from build123d import *

# Parameters (mm, degrees)
F0_R     = 11.2
F1_DEPTH = 7
F2_DEPTH = 7


with BuildPart() as f1:
    # F0 (on Top) → F1 (new body)
    with BuildSketch(Plane.XY):
        Polygon((7.778355, 38.276713), (-7.863495, 38.276713), (-14.210913, 26.261959), (-9.26244, 12.206962), (-15.820878, 2.988639), (-30.312402, -0.928071), (-37.037784, -12.402103), (-29.216858, -25.948344), (-15.638067, -25.437992), (-5.940319, -14.12499), (6.191501, -13.86279), (15.959934, -25.787275), (29.259428, -25.87461), (37.080354, -12.32837), (29.848981, -0.823968), (15.20276, 1.918027), (10.498676, 12.206962), (14.352468, 26.715346), align=None)
        with Locations((-20.96608, -12.037974)):
            Circle(F0_R, mode=Mode.SUBTRACT)
        Circle(F0_R, mode=Mode.SUBTRACT)
        with Locations((21.115096, -11.951939)):
            Circle(F0_R, mode=Mode.SUBTRACT)
        with Locations((0, 24.448412)):
            Circle(F0_R, mode=Mode.SUBTRACT)
    extrude(amount=F1_DEPTH)

    # F0 (on Top) → F2 (join)
    with BuildSketch(Plane.XY):
        Polygon((7.778355, 38.276713), (-7.863495, 38.276713), (-14.210913, 26.261959), (-9.26244, 12.206962), (-15.820878, 2.988639), (-30.312402, -0.928071), (-37.037784, -12.402103), (-29.216858, -25.948344), (-15.638067, -25.437992), (-5.940319, -14.12499), (6.191501, -13.86279), (15.959934, -25.787275), (29.259428, -25.87461), (37.080354, -12.32837), (29.848981, -0.823968), (15.20276, 1.918027), (10.498676, 12.206962), (14.352468, 26.715346), align=None)
        with Locations((-20.96608, -12.037974)):
            Circle(F0_R, mode=Mode.SUBTRACT)
        Circle(F0_R, mode=Mode.SUBTRACT)
        with Locations((21.115096, -11.951939)):
            Circle(F0_R, mode=Mode.SUBTRACT)
        with Locations((0, 24.448412)):
            Circle(F0_R, mode=Mode.SUBTRACT)
    extrude(amount=F2_DEPTH)


solid = f1.part
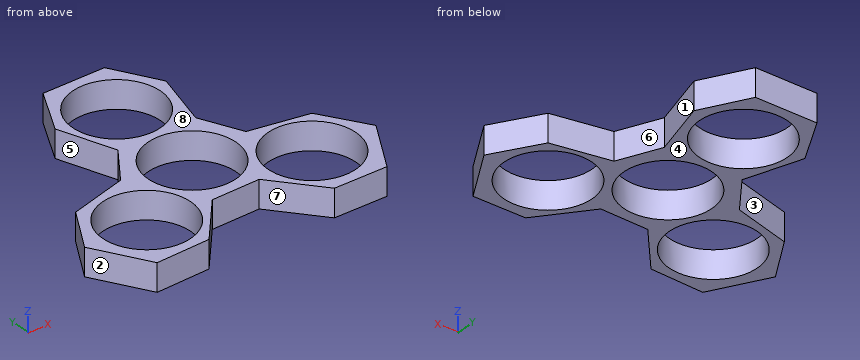
Read the model definition and answer for the solid it produces. Units are mm, in the model's axes. Face numbers are marked on the shaded views. A direction names the side the tool comes from. Round coordinates to 2 decimals unless told otherwise and drop trailing zeros. Write each loop counter-clockwise with the first axis right and the second up, starting at its lowest first coordinate (ties: lowest second). Pieces come first, ordered by that corner, then holes. Notation, with made-up numbers: (43, -34) - (56, -34) arc R17 ccw to (56, -3) - close; hole circle Ø1 at (41, -5). An arc over 180 degrees is marked (long way). Use a Markdown table: item, result.
(1) The part is cut by section A-A (y = -8.5). Write down the section's boundary in (x, z).
Reported:
| item | result |
|---|---|
| outline | (-34.75, 0) - (-31.59, 0) - (-31.59, 7) - (-34.75, 7) - close; (-10.34, 0) - (-7.29, 0) - (-7.29, 7) - (-10.34, 7) - close; (7.29, 0) - (10.46, 0) - (10.46, 7) - (7.29, 7) - close; (31.77, 0) - (34.67, 0) - (34.67, 7) - (31.77, 7) - close |
(2) The mould has two halves that part along Y. Classify the marked faces 1, 2, 3 and 4: released by +Y, released by -Y, zero draft, split by the parting line, or undercut.
Reported:
| item | result |
|---|---|
| face 1 | undercut |
| face 2 | released by -Y |
| face 3 | released by +Y |
| face 4 | zero draft |
(3) The part is cut by section B-B (x = -19). Write down the section's boundary in (y, z), then the cut area to 3 significant figures.
Reported:
| item | result |
|---|---|
| outline | (-25.56, 0) - (-23.06, 0) - (-23.06, 7) - (-25.56, 7) - close; (-1.01, 0) - (2.13, 0) - (2.13, 7) - (-1.01, 7) - close |
| area | 39.5 mm2 |
(4) The part is cut by section C-C (z = 2.25). Write down the section's boundary in (x, y) (1 decimal), then the cut area to 3 significant figures.
Reported:
| item | result |
|---|---|
| outline | (-37, -12.4) - (-29.2, -25.9) - (-15.6, -25.4) - (-5.9, -14.1) - (6.2, -13.9) - (16, -25.8) - (29.3, -25.9) - (37.1, -12.3) - (29.8, -0.8) - (15.2, 1.9) - (10.5, 12.2) - (14.4, 26.7) - (7.8, 38.3) - (-7.9, 38.3) - (-14.2, 26.3) - (-9.3, 12.2) - (-15.8, 3) - (-30.3, -0.9) - close; hole circle Ø22.4 at (-21, -12); hole circle Ø22.4 at (0, 0); hole circle Ø22.4 at (0, 24.4); hole circle Ø22.4 at (21.1, -12) |
| area | 831 mm2 |
(5) Straight lines are drawn through the part: line 1 along Y through (x, z) = (-2.5, 6); line 2 along X through (y, z) = (-17, 4.25); line 3 along X through (y, z) = (-19.5, 5.75). For each, find the intervals that lie inside material, in ascending order. Write a range as [from, to].
Reported:
| item | result |
|---|---|
| line 1 | [-14.05, -10.92], [10.92, 13.53], [35.37, 38.28] |
| line 2 | [-34.38, -31.01], [-10.93, -8.4], [8.76, 11.12], [31.11, 34.38] |
| line 3 | [-32.94, -29.32], [-12.61, -10.55], [10.81, 12.84], [29.39, 32.94] |
(6) The part is cut by section D-D (y = 7). Write down the section's boundary in (x, z), then the cut area to 3 significant figures.
Reported:
| item | result |
|---|---|
| outline | (-12.97, 0) - (-8.74, 0) - (-8.74, 7) - (-12.97, 7) - close; (8.74, 0) - (12.88, 0) - (12.88, 7) - (8.74, 7) - close |
| area | 58.5 mm2 |
(7) Each of these flat-tipped pins is pushed along its axis until it touches: pin 1 Ø1 at (y, z) = (-5, 5) entering from -X; pin 2 Ø8 at (x, y) = (13.5, 12.5) entering from -Z. Where does it stop, or does it pass through?
Reported:
| item | result |
|---|---|
| pin 1 | x = -32.99 |
| pin 2 | z = 0 |
(8) Which of the six approach directions +Z, -Z, +X, -X, +Y, -Y give full straight-line access (tool end or side, diameter ignored) to the marked faces 5, 6, 7 and 8?
Reported:
| item | result |
|---|---|
| face 5 | +Z, -Z, -X |
| face 6 | +Z, -Z, +X |
| face 7 | +Z, -Z, -Y |
| face 8 | +Z, +X, -X, +Y, -Y |
